```python
from build123d import *

# Parameters (mm, degrees)
F0_R     = 8.171292
F1_DEPTH = 12.7
F2_R     = 6.582327
F3_DEPTH = 127
F4_R     = 6.35
F5_SIZE  = 6.35


with BuildPart() as f1:
    # F0 (on Front) → F1 (new body, symmetric)
    with BuildSketch(Plane.XZ):
        with BuildLine():
            Line((0, 25.4), (0, 0))
            Line((0, 0), (76.2, 0))
            Line((76.2, 0), (76.2, -12.7))
            ThreePointArc((76.2, -12.7), (79.919744, -21.680256), (88.9, -25.4))
            Line((88.9, -25.4), (177.8, -25.4))
            Line((177.8, -25.4), (177.8, 0))
            Line((177.8, 0), (101.6, 0))
            ThreePointArc((101.6, 0), (92.619744, 3.719744), (88.9, 12.7))
            ThreePointArc((88.9, 12.7), (92.619744, 21.680256), (101.6, 25.4))
            Line((101.6, 25.4), (177.8, 25.4))
            Line((177.8, 25.4), (177.8, 50.8))
            Line((177.8, 50.8), (88.9, 50.8))
            ThreePointArc((88.9, 50.8), (79.919744, 47.080256), (76.2, 38.1))
            Line((76.2, 38.1), (76.2, 25.4))
            Line((76.2, 25.4), (0, 25.4))
        make_face()
        with Locations((12.7, 12.7)):
            Circle(F0_R, mode=Mode.SUBTRACT)
    extrude(amount=F1_DEPTH, both=True)

    # F2 (on face) → F3 (cut, symmetric)
    with BuildSketch(Plane.XY.offset(50.8)):
        with Locations((165.1, 0)):
            Circle(F2_R)
    extrude(amount=F3_DEPTH, both=True, mode=Mode.SUBTRACT)

    # F4
    f4_edges = [f1.edges().sort_by_distance(p)[0] for p in [
        (76.2, 0, 25.4),
        (76.2, 0, 0),
    ]]
    fillet(f4_edges, radius=F4_R)

    # F5
    f5_edges = [f1.edges().sort_by_distance(p)[0] for p in [
        (177.8, 12.7, 38.1),
        (177.8, -12.7, 38.1),
        (177.8, -12.7, -12.7),
        (177.8, 12.7, -12.7),
    ]]
    chamfer(f5_edges, length=F5_SIZE)


solid = f1.part
```
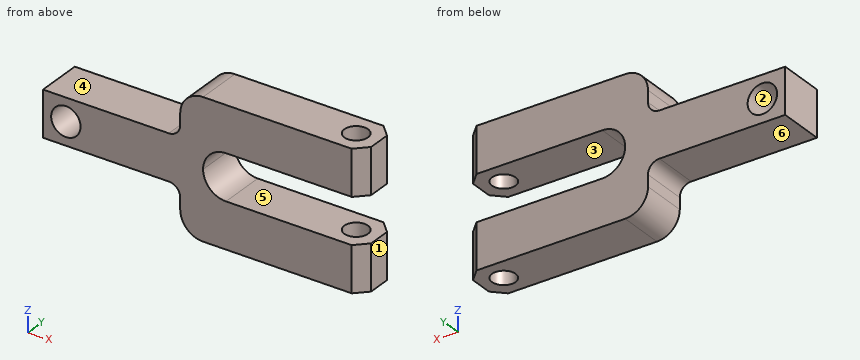
Geometry check sheet. Reference: the model listing, model coordinates, mm. Face numbers are marked on the shaded views. A direction names the side the tool comes from. Round coordinates to 2 decimals unless told otherwise and drop trailing zeros. Order: outer loops, then holes, each group sorted by start corner. A loop starts at its lowest first (then second) coordinate and runs counter-clockwise, first axis right, second up. Notation, with made-up numbers: (86, 71) -> (100, 71) arc R13 ccw to (100, 90) -> close; hole circle Ø4 at (70.25, 6). An arc over 180 degrees is marked (long way). Return JSON: item names as keys, results as strings. Group by question number.
Q1. Release check for a two-part mould opening along X. For the marked faces 1, 2 and 3 record: released by +X, released by -X, zero draft, split by the parting line, or undercut.
Q2. Tool access check on the marked faces 4, 5 and 6. Record the directions out of +Z, -Z, +X, -X, +Y, -Y that give a thin tool (end or side, any length) a straight path to the whole face; none if there is none.
Q3. Section check D-D, the plane z = -18.5. Record the boundary of the cut face in (x, y), plus the area to 3 significant figures.
Q4. Material ranges on probe 1 along Y at (x, z) = (165.1, 39.5); probe 2 along Z at (x, y) = (140, -6.25); probe 3 along Z at (x, y) = (12.7, -2.5), recorded low to high. Write a range as from..to.
Q5. Section check A-A, the plane x = 12.7. Record the boundary of the cut face in (y, z).
Q6. Gauge pin test, flat ends, axial feed: pin 1 (12.5 mm diameter, centred on x = 27, y = -5, fed in from -Z); pin 2 (6 mm diameter, centred on y = -2, z = 36, fed in from -X); pin 3 (3 mm diameter, centred on y = 6.5, z = 5, fed in from +X) (3 decimals); pin 4 (10 mm diameter, centred on x = 12.7, z = 12.7, fed in from -Y). Record the tip position at first contact, or that the pin passes through.
Q7. Section check B-B, the plane y = 0. Record the boundary of the cut face in (x, z), plus the area to 3 significant figures.
Q8. Section check C-C, the plane x = 165.1. Record the boundary of the cut face in (y, z), plus the area to 3 significant figures.
Numbers:
{
 "1": {"face 1": "released by +X", "face 2": "undercut", "face 3": "zero draft"},
 "2": {"face 4": "+Z, -X, +Y, -Y", "face 5": "+X, +Y, -Y", "face 6": "-Z, -X, +Y, -Y"},
 "3": {"outline": "(77.6, -12.7) -> (171.45, -12.7) -> (177.8, -6.35) -> (177.8, 6.35) -> (171.45, 12.7) -> (77.6, 12.7) -> close; hole circle Ø13.16 at (165.1, 0)", "area": "2,370 mm^2"},
 "4": {"probe 1": "-12.7..-6.58, 6.58..12.7", "probe 2": "-25.4..0, 25.4..50.8", "probe 3": "0..4.53, 20.87..25.4"},
 "5": {"outline": "(-12.7, 0) -> (12.7, 0) -> (12.7, 4.53) -> (-12.7, 4.53) -> close; (-12.7, 20.87) -> (12.7, 20.87) -> (12.7, 25.4) -> (-12.7, 25.4) -> close"},
 "6": {"pin 1": "z = 0", "pin 2": "x = 76.2", "pin 3": "x = 92.845", "pin 4": "through"},
 "7": {"outline": "(0, 0) -> (69.85, 0) arc R6.35 cw to (76.2, -6.35) -> (76.2, -12.7) arc R12.7 ccw to (88.9, -25.4) -> (158.52, -25.4) -> (158.52, 0) -> (101.6, 0) arc R12.7 cw to (101.6, 25.4) -> (158.52, 25.4) -> (158.52, 50.8) -> (88.9, 50.8) arc R12.7 ccw to (76.2, 38.1) -> (76.2, 31.75) arc R6.35 cw to (69.85, 25.4) -> (0, 25.4) -> close; (171.68, -25.4) -> (177.8, -25.4) -> (177.8, 0) -> (171.68, 0) -> close; (171.68, 25.4) -> (177.8, 25.4) -> (177.8, 50.8) -> (171.68, 50.8) -> close; hole circle Ø16.34 at (12.7, 12.7)", "area": "6,560 mm^2"},
 "8": {"outline": "(-12.7, -25.4) -> (-6.58, -25.4) -> (-6.58, 0) -> (-12.7, 0) -> close; (-12.7, 25.4) -> (-6.58, 25.4) -> (-6.58, 50.8) -> (-12.7, 50.8) -> close; (6.58, -25.4) -> (12.7, -25.4) -> (12.7, 0) -> (6.58, 0) -> close; (6.58, 25.4) -> (12.7, 25.4) -> (12.7, 50.8) -> (6.58, 50.8) -> close", "area": "622 mm^2"}
}
